```python
from build123d import *

# Parameters (mm, degrees)
SKETCH_R        = 4
PAD_DEPTH       = 1.2
SKETCH001_R     = 2.3
PAD001_DEPTH    = 1.8
SKETCH002_R     = 2.5
PAD002_DEPTH    = 1.2
CHAMFER_SIZE    = 0.5
CHAMFER001_SIZE = 0.19


with BuildPart() as part:
    # Sketch → Pad (new body)
    with BuildSketch(Plane.XY):
        Circle(SKETCH_R)
    extrude(amount=PAD_DEPTH)

    # Sketch001 → Pad001 (join)
    with BuildSketch(Plane.XY.offset(1.2)):
        Circle(SKETCH001_R)
    extrude(amount=PAD001_DEPTH)

    # Sketch002 → Pad002 (join)
    with BuildSketch(Plane.XY.offset(3)):
        Circle(SKETCH002_R)
    extrude(amount=-PAD002_DEPTH)

    # Chamfer
    chamfer_edges = [part.edges().sort_by_distance(p)[0] for p in [
        (-2.5, 0, 3),
        (-4, 0, 0),
    ]]
    chamfer(chamfer_edges, length=CHAMFER_SIZE)

    # Chamfer001
    chamfer001_edges = [part.edges().sort_by_distance(p)[0] for p in [
        (-2.5, 0, 1.8),
    ]]
    chamfer(chamfer001_edges, length=CHAMFER001_SIZE)


solid = part.part
```
Input: part model. Units: mm. Frame: model coordinates. A direction names the side the tool comes from. Give positions to 0.01 mm unless a question says otherwise; leave off trailing zeros. Order: outer loops, then holes, each group sorted by start corner. A loop starts at its lowest first (then second) coordinate and runs counter-clockwise, first axis right, second up. Notation, with made-up numbers: M -39,47.5 L -32,47.5 A12 ccw -32,56.5 Z; hole C 84.5,15 d1. An arc over 180 degrees is marked long. One line per question, with ' | ' between items. Start each with the question number.
1. Material intervals for probe 1 along Z at (x, y) = (2.5, -2.25); probe 2 along Z at (x, y) = (-1.75, 1.75); probe 3 along Y at (x, z) = (2.5, 0.8), sorted ascending. Write a range as [from, to].
2. First-contact query: pin 1 Ø1 at (y, z) = (-2, 1) entering from +X; pin 2 Ø2 at (x, y) = (3, 0.5) entering from +Z; pin 3 Ø1 at (x, z) = (3, 0.5) entering from -Y. Flat tips, straight axial feed; report the tip coordinate or a pass-through.
3. Section query C-C (z = 1.4). Return the cut outline in (x, y).
4. Access query for faces 1 (the face through (-0.54, -2.44, 2.25)), 2 (the face through (0, 0, 0)). Directions: +Z, -Z, +X, -X, +Y, -Y. A direction counts if a zero-diameter tool reaches every point of the face in a straight line with its end or side. Return the directions, or none.
5. Pull-direction query (Z, two-part tool) for faces 3 (the face through (-1.825, -1.4, 1.496)), 4 (the face through (-0.867, -3.905, 0.845)), 5 (the face through (0, 0, 3)); classes: released by +Z, released by -Z, zero draft, split by the parting line, or undercut.
6. Section query D-D (z = 2.75). Return the cut outline in (x, y).
Here are the results:
1) probe 1: [0, 1.2] | probe 2: [0, 1.2], [1.96, 2.53] | probe 3: [-3.12, 3.12]
2) pin 1: x = 3.71 | pin 2: z = 2.96 | pin 3: y = -3.12
3) outline: C 0,0 d4.6
4) face 1: +Z | face 2: -Z, +X, -X, +Y, -Y
5) face 3: undercut | face 4: zero draft | face 5: released by +Z
6) outline: C 0,0 d4.5
